from build123d import *

# Parameters (mm, degrees)
SKETCH1_R               = 3.3782
BOSS_EXTRUDE1_DEPTH     = 11.1125
SKETCH2_R               = 3.3655
CUT_EXTRUDE1_DEPTH      = 421.288113218
SKETCH3_R               = 3.3655
CUT_EXTRUDE2_DEPTH      = 421.177767573
SKETCH4_R               = 3.3655
CUT_EXTRUDE3_DEPTH      = 421.177767573
SKETCH5_R               = 3.3655
CUT_EXTRUDE4_DEPTH      = 421.177767573
CUT_EXTRUDE5_DEPTH      = 421.393634125
CUT_EXTRUDE5_DEPTH_BACK = 421.393634125
SKETCH6_R               = 3.3782
SKETCH7_W               = 18.18
SKETCH7_H               = 167.982857143
CUT_EXTRUDE6_DEPTH      = 693.582490434


with BuildPart() as part:
    # Sketch1 → Boss-Extrude1 (new body)
    with BuildSketch(Plane.XY):
        Polygon((-558.565, 76.762), (-458.235, 76.762), (-140.853700004, 76.762), (-84.973700004, 76.762), (-84.973700004, -12.5), (0, -12.5), (0, 216.1), (-63.5, 292.3), (-449.98, 292.3), (-627.78, 139.9), (-627.78, -12.5), (-558.565, -12.5), align=None)
        with Locations((-12.5, 203.6)):
            Circle(SKETCH1_R, mode=Mode.SUBTRACT)
    extrude(amount=BOSS_EXTRUDE1_DEPTH)

    # Sketch2 → Cut-Extrude1 (cut, through all)
    with BuildSketch(Plane(origin=(-305, 23.6125, -5.08), x_dir=(-1, 0, 0), z_dir=(0, 0, -1))):
        with Locations((288.9533823, 103.7145)):
            Circle(SKETCH2_R)
    extrude(amount=-CUT_EXTRUDE1_DEPTH, mode=Mode.SUBTRACT)

    # Sketch3 → Cut-Extrude2 (cut, through all)
    with BuildSketch(Plane(origin=(-305, 23.6125, -1.905), x_dir=(-1, 0, 0), z_dir=(0, 0, -1))):
        with Locations((141.846254523, 256.904809604)):
            Circle(SKETCH3_R)
    extrude(amount=-CUT_EXTRUDE2_DEPTH, mode=Mode.SUBTRACT)

    # Sketch4 → Cut-Extrude3 (cut, through all)
    with BuildSketch(Plane(origin=(-305, 23.6125, -1.905), x_dir=(-1, 0, 0), z_dir=(0, 0, -1))):
        with Locations((-48.26, 250.9075)):
            Circle(SKETCH4_R)
    extrude(amount=-CUT_EXTRUDE3_DEPTH, mode=Mode.SUBTRACT)

    # Sketch5 → Cut-Extrude4 (cut, through all)
    with BuildSketch(Plane(origin=(-305, 23.6125, -1.905), x_dir=(-1, 0, 0), z_dir=(0, 0, -1))):
        with Locations((-236.766660116, 257.207608298)):
            Circle(SKETCH5_R)
    extrude(amount=-CUT_EXTRUDE4_DEPTH, mode=Mode.SUBTRACT)

    # Sketch6 → Cut-Extrude5 (cut, two sides: drawn at the far end of the back side and taken through both)
    with BuildSketch(Plane(origin=(-305, 23.6125, 18.7325), x_dir=(1, 0, 0), z_dir=(0, 0, 1)).offset(-CUT_EXTRUDE5_DEPTH_BACK)):
        with Locations((-197.262125611, 186.926969688)):
            Circle(SKETCH6_R)
        with Locations((-33.209654284, 70.005387803)):
            Circle(SKETCH6_R)
        with Locations((-90.296950895, 152.235012548)):
            Circle(SKETCH6_R)
    extrude(amount=CUT_EXTRUDE5_DEPTH + CUT_EXTRUDE5_DEPTH_BACK, mode=Mode.SUBTRACT)

    # Sketch7 → Cut-Extrude6 (cut, through all)
    with BuildSketch(Plane.XY.offset(11.1125)):
        with Locations((-618.69, 71.491428572)):
            Rectangle(SKETCH7_W, SKETCH7_H)
    extrude(amount=-CUT_EXTRUDE6_DEPTH, mode=Mode.SUBTRACT)


solid = part.part
Here's how the part is built. I have some questions about the finished solid (model axes, mm). A direction names the side the tool comes from. Give positions to 0.01 mm unless a question says otherwise; leave off trailing zeros. Loops run counter-clockwise (first coordinate to the right, second up) from the corner with the lowest first, then second, coordinate; pieces in that order, holes last. Notation, with made-up numbers: (-33, 75) -> (-11, 75) arc R17 cw to (-11, 90) -> close; hole circle Ø10 at (58.25, 75). An arc over 180 degrees is marked (long way). Answer as a JSON object with one key per item and string values. Group by question number.
Item 1: Imagine slicing it at D-D on y = 252.5. Write out the boundary of the cut face in (x, z), then the cut area to 3 significant figures.
Item 2: On a 3-axis mill with a long thin cutter (end or side, diameter ignored), from which of +Z, -Z, +X, -X, +Y, -Y can I reach the whole of each face in a straight line? I mean faces 1 (the flat face through (-43, -12.5, 5)), 2 (the flat face through (-84.974, 33, 5)). Say none if no direction works.
Item 3: Will these pins go through, and if not, where does the flat tip stop? pin 1 (9 mm diameter, centred on x = -68.23, y = 280.82, fed in from -Z); pin 2 (5.5 mm diameter, centred on x = -256.74, y = 274.52, fed in from +Z); pin 3 (3.5 mm diameter, centred on x = -365.5, z = 4.5, fed in from -Y).
Item 4: Imagine slicing it at C-C on z = 9.25. Give the number of separate pieces and of enclosed holes in the cut face, then the cut area to 3 significant figures.
Item 5: I need wall thicknesses on L1, parallel to X at y = 62, z = 5.75 (3 decimals); L2, parallel to Y at x = -68, z = 10.5; L3, parallel to Y at x = -256.74, z = 5.25. Which ranges of each line are inside material? Lowest first, please.
Item 6: Thinking about a two-plate mould opening in X: for faces 3 (the flat face through (-558.565, 32, 5)), 4 (the flat face through (-254, 292.3, 5)), 5 (the flat face through (-528.67, 224.85, 5.48)), which applies, pulls with the +X half, pulls with the -X half, needs draft (parallel to the pull), parting line crosses it, or undercut?
Item 7: Imagine slicing it at A-A on y = 29. Write out the boundary of the cut face in (x, z) (1 decimal).
Item 8: Imagine slicing it at B-B on x = -163. Write out the boundary of the cut face in (y, z).
Answer list:
{
 "1": {"outline": "(-496.41, 0) -> (-30.33, 0) -> (-30.33, 11.11) -> (-496.41, 11.11) -> close", "area": "5,180 mm2"},
 "2": {"face 1": "+Z, -Z, +X, -X, -Y", "face 2": "+Z, -Z, -Y"},
 "3": {"pin 1": "stops at z = 0", "pin 2": "passes through", "pin 3": "stops at y = 76.76"},
 "4": {"separate pieces": "1", "enclosed holes": "8", "area": "130,000 mm2"},
 "5": {"L1": "x = -609.6 to -558.565, -84.974 to 0", "L2": "y = -12.5 to 277.46, 284.18 to 292.3", "L3": "y = 76.76 to 271.15, 277.89 to 292.3"},
 "6": {"face 3": "undercut", "face 4": "needs draft", "face 5": "pulls with the -X half"},
 "7": {"outline": "(-609.6, 0) -> (-558.6, 0) -> (-558.6, 11.1) -> (-609.6, 11.1) -> close; (-85, 0) -> (0, 0) -> (0, 11.1) -> (-85, 11.1) -> close"},
 "8": {"outline": "(76.76, 0) -> (292.3, 0) -> (292.3, 11.11) -> (76.76, 11.11) -> close"}
}
